```python
from build123d import *

# Parameters (mm, degrees)
SKETCH1_R           = 46.8
SKETCH1_W           = 5
SKETCH1_H           = 3.175
BOSS_EXTRUDE1_DEPTH = 3.175


with BuildPart() as part:
    # Sketch1 → Boss-Extrude1 (new body)
    with BuildSketch(Plane(origin=(0, 0, 0), x_dir=(1, 0, 0), z_dir=(0, 1, 0))):
        with Locations(Location((0, 0, 0), (0, 0, 270))):
            Circle(SKETCH1_R)
        with Locations((-12.5, 0)):
            Rectangle(SKETCH1_W, SKETCH1_H, mode=Mode.SUBTRACT)
        with Locations((12.5, 0)):
            Rectangle(SKETCH1_W, SKETCH1_H, mode=Mode.SUBTRACT)
    extrude(amount=BOSS_EXTRUDE1_DEPTH)


solid = part.part
```
The listing builds one solid part. Answer for the finished solid, in the listing's coordinates (mm). A direction names the side the tool comes from. Round coordinates to 2 decimals unless told otherwise and drop trailing zeros. Loops run counter-clockwise (first coordinate to the right, second up) from the corner with the lowest first, then second, coordinate; pieces in that order, holes last.
1) A cutting plane is placed at C-C on x = -13.5. Determine the outline of the cut face in (y, z) (1 decimal), plus the area to 3 significant figures.
Outcome:
outline: (0, -44.8) - (3.2, -44.8) - (3.2, -1.6) - (0, -1.6) - close; (0, 1.6) - (3.2, 1.6) - (3.2, 44.8) - (0, 44.8) - close
area: 274 mm2
2) For faces 1 (the face through (12, 2, -1.588)), 2 (the face through (1, 0, -1)), determine the directions among +Z, -Z, +X, -X, +Y, -Y from which every point of the face is accessible in a straight line to the end or side of a thin tool.
Outcome:
face 1: +Y, -Y
face 2: +Z, -Z, +X, -X, -Y
3) A cutting plane is placed at B-B on y = 1.85. Determine the outline of the cut face in (x, z), plus the area to 3 significant figures.
Outcome:
outline: circle Ø93.6 at (0, 0); hole (-15, -1.59) - (-10, -1.59) - (-10, 1.59) - (-15, 1.59) - close; hole (10, -1.59) - (15, -1.59) - (15, 1.59) - (10, 1.59) - close
area: 6,850 mm2
4) For a pull along Z with two mould halves and no side action, classify faces 3 (the face through (-10, 2, 0)), 4 (the face through (10, 2, 0)), 5 (the face through (-41.52, 1.565, 21.595)), 6 (the face through (1, 3.175, -1)) as released by +Z, released by -Z, zero draft, split by the parting line, or undercut.
Outcome:
face 3: undercut
face 4: undercut
face 5: split by the parting line
face 6: zero draft
5) Given P1, Ø1, axis at x = -13, y = 2, coming from the -Z side; P2, Ø1.5, axis at x = -27.5, y = 1.5, coming from the +Z side; P3, Ø1, axis at x = 13.5, y = 1.5, coming from the +Z side, each flat-ended and moving along its own axis, determine where each tip first touches the part or whether it passes through.
Outcome:
P1: stops at z = -45.1
P2: stops at z = 38.4
P3: stops at z = 44.96
6) A cutting plane is placed at A-A on z = 0. Determine the outline of the cut face in (x, y) (3 decimals).
Outcome:
outline: (-46.8, 0) - (-15, 0) - (-15, 3.175) - (-46.8, 3.175) - close; (-10, 0) - (10, 0) - (10, 3.175) - (-10, 3.175) - close; (15, 0) - (46.8, 0) - (46.8, 3.175) - (15, 3.175) - close
7) Consider line 1 (X direction, y = 2.05, z = -1.5); line 2 (Z direction, x = 14.5, y = 2.3); line 3 (Z direction, x = -1.5, y = 2.75). Determine where each line is inside the solid, lowest interval first.
Outcome:
line 1: x = -46.78 to -15, -10 to 10, 15 to 46.78
line 2: z = -44.5 to -1.59, 1.59 to 44.5
line 3: z = -46.78 to 46.78
8) A cutting plane is placed at D-D on z = 22. Determine the outline of the cut face in (x, y) (3 decimals), plus the area to 3 significant figures.
Outcome:
outline: (-41.307, 0) - (41.307, 0) - (41.307, 3.175) - (-41.307, 3.175) - close
area: 262 mm2
